from build123d import *

# Parameters (mm, degrees)
ESQUISSE1_W             = 10
ESQUISSE1_H             = 30
BOSS_EXTRU_1_DEPTH      = 14
ESQUISSE2_W             = 3
ESQUISSE2_H             = 30
BOSS_EXTRU_2_DEPTH      = 10
ESQUISSE3_R             = 1.625
ENL_V_MAT_EXTRU_1_DEPTH = 4
ENL_V_MAT_EXTRU_2_DEPTH = 31


with BuildPart() as part:
    # Esquisse1 → Boss.-Extru.1 (new body)
    with BuildSketch(Plane.XY):
        with Locations((5, -15)):
            Rectangle(ESQUISSE1_W, ESQUISSE1_H)
    extrude(amount=BOSS_EXTRU_1_DEPTH)

    # Esquisse2 → Boss.-Extru.2 (add)
    with BuildSketch(Plane(origin=(10, 0, 0), x_dir=(0, 0, -1), z_dir=(1, 0, 0))):
        with Locations((-1.5, -15)):
            Rectangle(ESQUISSE2_W, ESQUISSE2_H)
    extrude(amount=BOSS_EXTRU_2_DEPTH)

    # Esquisse3 → Enlèv. mat.-Extru.1 (cut, through all)
    with BuildSketch(Plane.XY.offset(3)):
        with Locations((15, -5)):
            Circle(ESQUISSE3_R)
        with Locations((15, -25)):
            Circle(ESQUISSE3_R)
    extrude(amount=-ENL_V_MAT_EXTRU_1_DEPTH, mode=Mode.SUBTRACT)

    # Esquisse4 → Enlèv. mat.-Extru.2 (cut, through all)
    with BuildSketch(Plane.XZ.offset(30)):
        Polygon((10, 14), (0, 14), (0, 13.85), align=None)
    extrude(amount=-ENL_V_MAT_EXTRU_2_DEPTH, mode=Mode.SUBTRACT)


solid = part.part
Verification items for the finished model (mm, model axes). A direction names the side the tool comes from. Round coordinates to 2 decimals unless told otherwise and drop trailing zeros. Order: outer loops, then holes, each group sorted by start corner. A loop starts at its lowest first (then second) coordinate and runs counter-clockwise, first axis right, second up. Notation, with made-up numbers: (86, 77.5) -> (107, 77.5) arc R12 cw to (107, 83.5) -> close; hole circle Ø9 at (-35, -15.5). An arc over 180 degrees is marked (long way). Put each result on its own line as item: value.
1) Section check C-C (z = 1.5). Record the cut outline in (x, y) (3 decimals), then the cut area to 3 significant figures.
Final values:
outline: (0, -30) -> (20, -30) -> (20, 0) -> (0, 0) -> close; hole circle Ø3.25 at (15, -25); hole circle Ø3.25 at (15, -5)
area: 583 mm^2
2) Mould release check, pull along Y, two halves, no side actions. Record for faces 3 (the cylindrical face through (16.5, -25.62, 1.52)), 4 (the flat face through (0, -15, 7)), 5 (the cylindrical face through (16.55, -4.51, 1.52)), 6 (the flat face through (8, 0, 6)): +Y half, -Y half, draft (parallel to the pull), parting line (faces both ways), or undercut.
Final values:
face 3: undercut
face 4: draft
face 5: undercut
face 6: +Y half
3) Section check A-A (y = -25). Record the cut outline in (x, z) (3 decimals).
Final values:
outline: (0, 0) -> (13.375, 0) -> (13.375, 3) -> (10, 3) -> (10, 14) -> (0, 13.85) -> close; (16.625, 0) -> (20, 0) -> (20, 3) -> (16.625, 3) -> close
4) Section check B-B (x = 15). Record the cut outline in (y, z) (3 decimals), then the cut area to 3 significant figures.
Final values:
outline: (-30, 0) -> (-26.625, 0) -> (-26.625, 3) -> (-30, 3) -> close; (-23.375, 0) -> (-6.625, 0) -> (-6.625, 3) -> (-23.375, 3) -> close; (-3.375, 0) -> (0, 0) -> (0, 3) -> (-3.375, 3) -> close
area: 70.5 mm^2
5) Depth check by flat-ended pin: pin 1 (1 mm diameter, centred on x = 4, z = 7.5, fed in from +Y); pin 2 (2 mm diameter, centred on y = -16, z = 9, fed in from +X); pin 3 (5 mm diameter, centred on x = 7, y = -10, fed in from +Z); pin 4 (4 mm diameter, centred on x = 15, y = -25, fed in from +Z). Enter the tip coordinate at first touch or a pass-through.
Final values:
pin 1: stops at y = 0
pin 2: stops at x = 10
pin 3: stops at z = 13.99
pin 4: stops at z = 3
6) Set-up check for faces 1 (the flat face through (10, -15, 8)), 2 (the flat face through (10, -15, 0)): record each of +Z, -Z, +X, -X, +Y, -Y from which the full face is reachable in a straight line by a thin tool's end or side.
Final values:
face 1: +Z, +X, +Y, -Y
face 2: -Z, +X, -X, +Y, -Y
7) Section check D-D (y = -4). Record the cut outline in (x, z), then the cut area to 3 significant figures.
Final values:
outline: (0, 0) -> (13.72, 0) -> (13.72, 3) -> (10, 3) -> (10, 14) -> (0, 13.85) -> close; (16.28, 0) -> (20, 0) -> (20, 3) -> (16.28, 3) -> close
area: 162 mm^2
8) Material ranges on line 1 (Y direction, x = 15, z = 1.2) (3 decimals); line 2 (Z direction, x = 17, y = -7); line 3 (X direction, y = -23.5, z = 5.75), recorded low to high.
Final values:
line 1: y = -30 to -26.625, -23.375 to -6.625, -3.375 to 0
line 2: z = 0 to 3
line 3: x = 0 to 10
